Source: CAD feature listing. Evaluate the final solid. Frame: model axes, mm. A direction names the side the tool comes from. Coordinates: 2 decimals unless noted, no trailing zeros. Order: outer loops, then holes, each group sorted by start corner. A loop starts at its lowest first (then second) coordinate and runs counter-clockwise, first axis right, second up. Notation, with made-up numbers: (60, 85) - (92, 85) arc R18 cw to (92, 91) - close; hole circle Ø10 at (71.25, -13). An arc over 180 degrees is marked (long way). One line per question, with ' | ' between items. Start each with the question number.
(1) Contact query for flat-ended pins moving along their axis: P1, Ø2, axis at x = -2, y = 9.5, coming from the +Z side; P2, Ø1, axis at y = 1.5, z = -7, coming from the +X side; P3, Ø3, axis at x = -8, y = 5, coming from the +Z side; P4, Ø5, axis at x = 1.5, y = -2, coming from the -Z side. Output: stop coordinate, or through.
(2) Access query for faces 4 (the cylindrical face through (-1.494, 11.267, 5.86)), 5 (the cylindrical face through (-8.04, 7.81, 1.73)). Directions: +Z, -Z, +X, -X, +Y, -Y. A direction counts if a zero-diameter tool reaches every point of the face in a straight line with its end or side. Return the directions, or none.
(3) Section A-A (z = 0). Return the cut outline in (x, y) (3 decimals).
(4) Line query: line 1 along Y through (x, z) = (2, 0); line 2 along Z through (x, y) = (2.25, -10); line 3 along X through (y, z) = (6.5, -7.5). Output: solid intervals per line, ascending.
(5) Draft query along Z for faces 1 (the flat face through (-12.7, 8, -3)), 2 (the flat face through (-3.5, -8, 2)), 3 (the cylindrical face through (-8.082, 15.497, 3.441)). Return one class per face: +Z half, -Z half, draft (parallel to the pull), parting line (faces both ways), or undercut.
(6) Section C-C (x = -0.25). Return the cut outline in (y, z), then the cut area to 3 significant figures.
(7) Section D-D (x = -7.5). Return the cut outline in (y, z) (3 decimals).
from build123d import *

# Parameters (mm, degrees)
SKETCH2_R           = 12.7
SKETCH2_R_2         = 11.412
BOSS_EXTRUDE1_DEPTH = 9.85


with BuildPart() as part:
    # Sketch1 → Revolve1 (revolve)
    with BuildSketch(Plane.XY, mode=Mode.PRIVATE) as revolve1_sk:
        with BuildLine():
            Line((-3.5, 8), (-3.5, 11.412))
            Line((-3.5, 11.412), (-6.35, 11.412))
            Line((-6.35, 11.412), (-6.35, 15.875))
            Line((-6.35, 15.875), (-9.767060633, 15.875))
            Line((-9.767060633, 15.875), (-11.600147737, 12.7))
            ThreePointArc((-11.600147737, 12.7), (-12.065, 12.235147737), (-12.7, 12.065))
            Line((-12.7, 12.065), (-12.7, 8))
            Line((-12.7, 8), (-3.5, 8))
        make_face()
    revolve(revolve1_sk.sketch.rotate(Axis((0, 0, 0), (-1, 0, 0)), 90), axis=Axis((0, 0, 0), (-1, 0, 0)))

    # Sketch2 → Boss-Extrude1 (add)
    with BuildSketch(Plane(origin=(-6.35, 0, 0), x_dir=(0, 0, -1), z_dir=(1, 0, 0))):
        with Locations(Location((0, 0, 0), (0, 0, 180))):
            Circle(SKETCH2_R)
        with Locations(Location((0, 0, 0), (0, 0, 180))):
            Circle(SKETCH2_R_2, mode=Mode.SUBTRACT)
    extrude(amount=BOSS_EXTRUDE1_DEPTH)


solid = part.part
Response values:
1) P1: stops at z = 9.44 | P2: passes through | P3: stops at z = 15.48 | P4: stops at z = -12.7
2) face 4: +X | face 5: +X, -X
3) outline: (-12.7, -12.065) arc R1.27 cw to (-11.6, -12.7) - (-9.767, -15.875) - (-6.35, -15.875) - (-6.35, -12.7) - (3.5, -12.7) - (3.5, -11.412) - (-3.5, -11.412) - (-3.5, -8) - (-12.7, -8) - close; (-12.7, 8) - (-3.5, 8) - (-3.5, 11.412) - (3.5, 11.412) - (3.5, 12.7) - (-6.35, 12.7) - (-6.35, 15.875) - (-9.767, 15.875) - (-11.6, 12.7) arc R1.27 cw to (-12.7, 12.065) - close
4) line 1: y = -12.7 to -11.41, 11.41 to 12.7 | line 2: z = -7.83 to -5.5, 5.5 to 7.83 | line 3: x = -12.7 to -3.5
5) face 1: draft | face 2: undercut | face 3: parting line
6) outline: circle Ø25.4 at (0, 0); hole circle Ø22.82 at (0, 0) | area: 97.6 mm²
7) outline: circle Ø31.75 at (0, 0); hole circle Ø16 at (0, 0)
